Could you check a few things on this model? Use its own coordinates, in mm. A direction names the side the tool comes from. Give positions to 0.01 mm unless a question says otherwise; leave off trailing zeros. Loops run counter-clockwise (first coordinate to the right, second up) from the corner with the lowest first, then second, coordinate; pieces in that order, holes last. Notation, with made-up numbers: (45, 52) - (61, 52) arc R25 cw to (61, 68) - close; hole circle Ø10 at (6.5, -8). An arc over 180 degrees is marked (long way). Write each question's results on one line, items separated by ' | '. Start each with the question number.
Autodesk Inventor part; units mm, degrees
ref_plane "YZ Plane" through (0, 0, 0) normal (1, 0, 0) x (0, 1, 0)
ref_plane "XZ Plane" through (0, 0, 0) normal (0, 1, 0) x (-1, 0, 0)
ref_plane "XY Plane" through (0, 0, 0) normal (0, 0, 1) x (1, 0, 0)
sketch "Sketch1" plane through (0, 0, 0) normal (0, 0, 1) x (1, 0, 0)
  line L0 (-10, -142.3192) -> (-10, -139.3192)
  line L1 (-10, -139.3192) -> (10, -139.3192)
  line L2 (10, -139.3192) -> (10, -142.3192)
  line L3 (10, -142.3192) -> (25, -142.3192)
  line L4 (25, -142.3192) -> (25, -139.3192)
  line L5 (25, -139.3192) -> (22, -139.3192)
  line L6 (22, -139.3192) -> (22, -109.3192)
  line L7 (22, -109.3192) -> (25, -109.3192)
  line L8 (25, -109.3192) -> (25, -79.3192)
  line L9 (25, -79.3192) -> (22, -79.3192)
  line L10 (22, -79.3192) -> (22, -49.3192)
  line L11 (22, -49.3192) -> (25, -49.3192)
  line L12 (25, -49.3192) -> (64.7409, 7.7563)
  line L13 (64.7409, 7.7563) -> (64.7409, 124.1392)
  arc A0 (64.7409, 124.1392) -> (58.7409, 130.1392) centre (58.7409, 124.1392) ccw
  line L14 (58.7409, 130.1392) -> (41.2562, 130.1392)
  arc A1 (12.5221, 134.8494) -> (41.2562, 130.1392) centre (41.2562, 220.1392) ccw
  arc A2 (12.5221, 134.8494) -> (-12.5221, 134.8494) centre (0, 97.6808) ccw
  arc A3 (-41.2562, 130.1392) -> (-12.5221, 134.8494) centre (-41.2562, 220.1392) ccw
  line L15 (-41.2562, 130.1392) -> (-58.7409, 130.1392)
  arc A4 (-58.7409, 130.1392) -> (-64.7409, 124.1392) centre (-58.7409, 124.1392) ccw
  line L16 (-64.7409, 124.1392) -> (-64.7409, 7.7563)
  line L17 (-64.7409, 7.7563) -> (-25, -49.3192)
  line L18 (-25, -49.3192) -> (-22, -49.3192)
  line L19 (-22, -49.3192) -> (-22, -79.3192)
  line L20 (-22, -79.3192) -> (-25, -79.3192)
  line L21 (-25, -79.3192) -> (-25, -109.3192)
  line L22 (-25, -109.3192) -> (-22, -109.3192)
  line L23 (-22, -109.3192) -> (-22, -139.3192)
  line L24 (-22, -139.3192) -> (-25, -139.3192)
  line L25 (-25, -139.3192) -> (-25, -142.3192)
  line L26 (-25, -142.3192) -> (-10, -142.3192)
  circle A5 centre (-50, 115.7563) radius 3.25
  circle A6 centre (50, 115.7563) radius 3.25
  circle A7 centre (20.018, 7.7563) radius 3.25
  circle A8 centre (-20.018, 7.7563) radius 3.25
  circle A9 centre (-28.3016, 116.7669) radius 4
  circle A10 centre (-20.018, 32.7797) radius 4
  circle A11 centre (20.018, 32.7797) radius 4
  circle A12 centre (28.3016, 116.7669) radius 4
  line L27 (32.1264, 90.1891) -> (26.4217, 48.2224)
  arc A13 (14.6157, 49.8272) -> (26.4217, 48.2224) centre (20.5187, 49.0248) ccw
  line L28 (14.6157, 49.8272) -> (20.3204, 91.794)
  arc A14 (32.1264, 90.1891) -> (20.3204, 91.794) centre (26.2234, 90.9915) ccw
  line L29 (-20.3204, 91.794) -> (-14.6157, 49.8272)
  arc A15 (-26.4217, 48.2224) -> (-14.6157, 49.8272) centre (-20.5187, 49.0248) ccw
  line L30 (-26.4217, 48.2224) -> (-32.1264, 90.1891)
  arc A16 (-20.3204, 91.794) -> (-32.1264, 90.1891) centre (-26.2234, 90.9915) ccw
  circle A17 centre (50, 115.7563) radius 6.25
  circle A18 centre (-50, 115.7563) radius 6.25
  circle A19 centre (20.018, 7.7563) radius 6.25
  circle A20 centre (-20.018, 7.7563) radius 6.25
  point P0 (0, 0)
  dimension "d0" = 3
  dimension "d1" = 3
  dimension "d2" = 3
  dimension "d3" = 3
extrude "Extrusion1" add sketch "Sketch1" along normal blind 6 contours L26 L25 L24 L23 L22 L21 L20 L19 L18 L17 L16 A4 L15 A3 A2 A1 L14 A0 L13 L12 L11 L10 L9 L8 L7 L6 L5 L4 L3 L2 L1 L0
properties part number "Camera stand plate base"
Q1. I'm going to push flat-ended pins straight in: pin 1 Ø1.5 at (x, z) = (-6, 1) entering from -Y; pin 2 Ø1 at (x, z) = (-39.5, 1) entering from -Y; pin 3 Ø8 at (x, y) = (-27, 49.5) entering from -Z; pin 4 Ø11 at (x, y) = (-20.02, 7.76) entering from +Z. Where does each tip first touch, or does it pass through?
Q2. Which directions (+Z, -Z, +X, -X, +Y, -Y) give clear straight access to the entire face, cutting with the end or side of a thin tool? Please do faces 1 (the face through (25, -95, 3)), 2 (the face through (0, -139.319, 3)), 3 (the face through (50, 130.139, 3)).
Q3. I want a section at B-B, the plane y = 65.5. List the corners of the cut face in (x, z) for me, then the cut area to 3 significant figures.
Q4. If we mould it in two halves opening along Y, with no side actions, what happens to faces 4 (the face through (15.06, 11.56, 2.96)), 5 (the face through (62.937, 128.428, 2.958)), 6 (the face through (-1, 30, 6)), 7 (the face through (26.9, 96.91, 2.96))? For each: +Y half, -Y half, draft (parallel to the pull), parting line (faces both ways), or undercut.
Q5. I need wall thicknesses on L1, parallel to Y at x = -25.5, z = 1.75; L2, parallel to Y at x = 22.5, z = 4.4; L3, parallel to X at y = 121, z = 3.55. Which ranges of each line are inside material? Lowest first, please. Write a range as from..to.
Q6. I want a section at C-C, the plane z = 4.8. State how many separate pieces and enclosed holes the cut face has, then the cut area to 3 significant figures.
Q7. I want a section at A-A, the plane x = 50. List the corners of the cut face in (y, z) for me, then the cut area to 3 significant figures.
Conclusion:
1) pin 1: y = -139.32 | pin 2: y = -29.21 | pin 3: z = 0 | pin 4: through
2) face 1: +Z, -Z, +X, -Y | face 2: +Z, -Z, -Y | face 3: +Z, -Z, +X, +Y
3) outline: (-64.74, 0) - (-28.77, 0) - (-28.77, 6) - (-64.74, 6) - close; (-16.75, 0) - (16.75, 0) - (16.75, 6) - (-16.75, 6) - close; (28.77, 0) - (64.74, 0) - (64.74, 6) - (28.77, 6) - close | area: 633 mm^2
4) face 4: undercut | face 5: +Y half | face 6: draft | face 7: undercut
5) L1: -48.6..4.75, 10.76..45.76, 96.9..113.91, 119.62..131.53 | L2: -142.32..-139.32, -109.32..-79.32, -49.32..2.02, 13.49..29.64, 35.92..43.41, 95.64..132.12 | L3: -64.74..-53.4, -46.6..46.6, 53.4..64.74
6) separate pieces: 1 | enclosed holes: 10 | area: 23,500 mm^2
7) outline: (-13.41, 0) - (109.51, 0) - (109.51, 6) - (-13.41, 6) - close; (122.01, 0) - (130.14, 0) - (130.14, 6) - (122.01, 6) - close | area: 786 mm^2
